The listing builds one solid part. Answer for the finished solid, in the listing's coordinates (mm). A direction names the side the tool comes from. Give positions to 0.01 mm unless a question says otherwise; leave off trailing zeros. Loops run counter-clockwise (first coordinate to the right, second up) from the corner with the lowest first, then second, coordinate; pieces in that order, holes last. Notation, with made-up numbers: (52.5, 30) - (105.5, 30) arc R18 ccw to (105.5, 41) - close; hole circle Ø5 at (1.5, -16). An arc over 180 degrees is marked (long way). Answer as CSV lines item,"result". Start each with the question number.
1) A cutting plane is placed at B-B (y = -6.45). Determine the outline of the cut face in (x, z), and give its area (3 significant figures).
2) A cutting plane is placed at D-D (x = 0). Determine the outline of the cut face in (y, z), and give its area (3 significant figures).
3) Flat-ended cylindrical pins translate along their axes: pin 1 (1 mm diameter, centred on x = -1.5, z = 2.5, fed in from +Y); pin 2 (4 mm diameter, centred on x = 0, z = 5, fed in from +Y); pin 3 (3 mm diameter, centred on x = -5.25, y = -1.25, fed in from -Z); pin 4 (1 mm diameter, centred on y = 1, z = 8, fed in from -X). Find the tip coordinate at first contact, or state that the pin passes through.
4) For a pull along Y with two mould halves and no side action, classify faces 1 (the face through (-7.72, -7.95, 5.07)), 2 (the face through (0, 2, 0)), 3 (the face through (7.78, -7.95, 5.07)), 4 (the face through (-9.088, 11.279, 8.798)) as pulls with the +Y half, pulls with the -Y half, needs draft (parallel to the pull), parting line crosses it, or undercut.
5) Find the intervals of material crossed by line 1 along Z through (x, y) = (0, 10.4); line 2 along Z through (x, y) = (6.85, -6.45); line 3 along Y through (x, z) = (2.75, 4.5), in increasing order.
6) For faces 5 (the face through (0, 11.45, 9)), 6 (the face through (5.25, -8, 4)), 7 (the face through (0.694, 9.864, 1.876)), determine the directions among +Z, -Z, +X, -X, +Y, -Y from which every point of the face is accessible in a straight line to the end or side of a thin tool.
7) A cutting plane is placed at C-C (x = 6.75). Determine the outline of the cut face in (y, z), and give its area (3 significant figures).
8) A cutting plane is placed at A-A (z = 5). Determine the outline of the cut face in (x, y), and give its area (3 significant figures).
```python
from build123d import *

# Parameters (mm, degrees)
EXTRUDE_1_DEPTH     = 10
SKETCH_2_R          = 3.2
CUT_EXTRUDE_1_DEPTH = 2.6
SKETCH_3_R          = 1.5
CUT_EXTRUDE_2_DEPTH = 26.521608492
SKETCH_4_R          = 1
CUT_EXTRUDE_3_DEPTH = 19.334802971
FILLET_1_R          = 3
CHAMFER_1_SIZE      = 0.6


with BuildPart() as part:
    # ｽｹｯﾁ1 → ﾎﾞｽ - 押し出し1 (new body)
    with BuildSketch(Plane.XY):
        Polygon((-10.25, 11.45), (-10.25, -11.45), (-5.25, -11.45), (-5.25, -1.25), (5.25, -1.25), (5.25, -11.45), (10.25, -11.45), (10.25, 11.45), align=None)
    extrude(amount=EXTRUDE_1_DEPTH)

    # ｽｹｯﾁ2 → ｶｯﾄ - 押し出し1 (cut)
    with BuildSketch(Plane(origin=(0, 11.45, 0), x_dir=(1, 0, 0), z_dir=(0, 1, 0))):
        with Locations(Location((0, -5, 0), (0, 0, 180))):
            Circle(SKETCH_2_R)
    extrude(amount=-CUT_EXTRUDE_1_DEPTH, mode=Mode.SUBTRACT)

    # ｽｹｯﾁ3 → ｶｯﾄ - 押し出し2 (cut, through all)
    with BuildSketch(Plane(origin=(10.25, 0, 0), x_dir=(0, 0, -1), z_dir=(1, 0, 0))):
        with Locations(Location((-5, -6.45, 0), (0, 0, 90))):
            Circle(SKETCH_3_R)
    extrude(amount=-CUT_EXTRUDE_2_DEPTH, mode=Mode.SUBTRACT)

    # ｽｹｯﾁ4 → ｶｯﾄ - 押し出し3 (cut, through all)
    with BuildSketch(Plane.XY.offset(10)):
        with Locations((5.25, -1.25)):
            Circle(SKETCH_4_R)
        with Locations((-5.25, -1.25)):
            Circle(SKETCH_4_R)
    extrude(amount=-CUT_EXTRUDE_3_DEPTH, mode=Mode.SUBTRACT)

    # ﾌｨﾚｯﾄ1
    fillet_1_edges = [part.edges().sort_by_distance(p)[0] for p in [
        (-10.25, 0, 0),
        (10.25, 0, 0),
        (10.25, 0, 10),
        (-10.25, 0, 10),
    ]]
    fillet(fillet_1_edges, radius=FILLET_1_R)

    # 面取り1
    chamfer_1_edges = [part.edges().sort_by_distance(p)[0] for p in [
        (3.2, 11.45, 5),
        (0, 11.45, 0),
        (-10.25, 11.45, 5),
        (0, 11.45, 10),
        (10.25, 11.45, 5),
        (9.371320344, 11.45, 9.121320344),
        (9.371320344, 11.45, 0.878679656),
        (-9.371320344, 11.45, 9.121320344),
        (-9.371320344, 11.45, 0.878679656),
    ]]
    chamfer(chamfer_1_edges, length=CHAMFER_1_SIZE)


solid = part.part
```
Ans:
1,outline,"(-10.25, 3) arc R3 ccw to (-7.25, 0) - (-5.25, 0) - (-5.25, 3.5) - (-10.25, 3.5) - close; (-10.25, 6.5) - (-5.25, 6.5) - (-5.25, 10) - (-7.25, 10) arc R3 ccw to (-10.25, 7) - close; (5.25, 0) - (7.25, 0) arc R3 ccw to (10.25, 3) - (10.25, 3.5) - (5.25, 3.5) - close; (5.25, 6.5) - (10.25, 6.5) - (10.25, 7) arc R3 ccw to (7.25, 10) - (5.25, 10) - close"
1,area,"62.3 mm2"
2,outline,"(-1.25, 0) - (10.85, 0) - (11.45, 0.6) - (11.45, 1.2) - (10.85, 1.8) - (8.85, 1.8) - (8.85, 8.2) - (10.85, 8.2) - (11.45, 8.8) - (11.45, 9.4) - (10.85, 10) - (-1.25, 10) - close"
2,area,"110 mm2"
3,pin 1,"y = 11.07"
3,pin 2,"y = 8.85"
3,pin 3,"z = 0"
3,pin 4,"x = -10.21"
4,face 1,"undercut"
4,face 2,"needs draft"
4,face 3,"undercut"
4,face 4,"pulls with the +Y half"
5,line 1,"0 to 1.8, 8.2 to 10"
5,line 2,"0 to 3.5, 6.5 to 10"
5,line 3,"-1.25 to 8.85"
6,face 5,"+Z, -Z, +X, -X, +Y"
6,face 6,"+Z, -Z, -Y"
6,face 7,"+Y"
7,outline,"(-11.45, 0) - (10.85, 0) - (11.45, 0.6) - (11.45, 9.4) - (10.85, 10) - (-11.45, 10) - close; hole circle Ø3 at (-6.45, 5)"
7,area,"222 mm2"
8,outline,"(-10.25, -11.45) - (-5.25, -11.45) - (-5.25, -7.95) - (-10.25, -7.95) - close; (-10.25, -4.95) - (-5.25, -4.95) - (-5.25, -2.25) arc R1 cw (long way) to (-4.25, -1.25) - (4.25, -1.25) arc R1 cw (long way) to (5.25, -2.25) - (5.25, -4.95) - (10.25, -4.95) - (10.25, 10.85) - (9.65, 11.45) - (3.8, 11.45) - (3.2, 10.85) - (3.2, 8.85) - (-3.2, 8.85) - (-3.2, 10.85) - (-3.8, 11.45) - (-9.65, 11.45) - (-10.25, 10.85) - close; (5.25, -11.45) - (10.25, -11.45) - (10.25, -7.95) - (5.25, -7.95) - close"
8,area,"310 mm2"
